Autodesk Inventor part; units mm, degrees
ref_plane "YZ Plane" through (0, 0, 0) normal (1, 0, 0) x (0, 1, 0)
ref_plane "XZ Plane" through (0, 0, 0) normal (0, 1, 0) x (-1, 0, 0)
ref_plane "XY Plane" through (0, 0, 0) normal (0, 0, 1) x (1, 0, 0)
sketch "Sketch1" plane through (0, 0, 0) normal (0, 1, 0) x (-1, 0, 0)
  line L0 (115, 92.5) -> (-115, 92.5)
  line L1 (-115, 92.5) -> (-115, -92.5)
  line L2 (-115, -92.5) -> (115, -92.5)
  line L3 (115, -92.5) -> (115, 92.5)
  point P0 (0, 0)
  dimension "d0" = 230
  dimension "d1" = 185
  dimension "d2" = 115
  dimension "d3" = 92.5
extrude "Extrusion1" add sketch "Sketch1" along normal blind 5
sketch "Sketch2" plane through (0, 0, 0) normal (0, -1, 0) x (1, 0, 0)
  line L0 (110, 87.5) -> (-110, 87.5)
  line L1 (-110, 87.5) -> (-110, -87.5)
  line L2 (-110, -87.5) -> (110, -87.5)
  line L3 (110, -87.5) -> (110, 87.5)
  line L4 (-115, 92.5) -> (115, 92.5)
  line L5 (-115, -92.5) -> (-115, 92.5)
  line L6 (115, -92.5) -> (-115, -92.5)
  line L7 (115, 92.5) -> (115, -92.5)
  line L8 (115, 92.5) -> (-115, 92.5)
  line L9 (-115, 92.5) -> (-115, -92.5)
  line L10 (-115, -92.5) -> (115, -92.5)
  line L11 (115, -92.5) -> (115, 92.5)
  point P0 (0, 0)
  dimension "d109" = 5
  dimension "d110" = 5
  dimension "d111" = 5
  dimension "d112" = 5
extrude "Extrusion2" add sketch "Sketch2" along normal blind 17.5
sketch "Sketch3" plane through (0, 5, 0) normal (0, 1, 0) x (1, 0, 0)
  circle A0 centre (-50, 0) radius 15.5
  point P0 (0, 0)
  dimension "d12" = 31
  dimension "d13" = 50
extrude "Extrusion3" cut sketch "Sketch3" against normal through all
sketch "Sketch4" plane through (0, 5, 0) normal (0, 1, 0) x (1, 0, 0)
  circle A0 centre (-50, 0) radius 15.5
  line L0 (-115, -92.5) -> (115, -92.5)
  line L1 (115, -92.5) -> (115, 92.5)
  line L2 (115, 92.5) -> (-115, 92.5)
  line L3 (-115, 92.5) -> (-115, -92.5)
  circle A1 centre (-97.5, -75) radius 7.5
  circle A2 centre (-97.5, 75) radius 7.5
  circle A3 centre (97.5, -75) radius 7.5
  circle A4 centre (97.5, 75) radius 7.5
  circle A5 centre (-97.5, -75) radius 8.5
  circle A6 centre (-97.5, 75) radius 8.5
  circle A7 centre (97.5, 75) radius 8.5
  circle A8 centre (97.5, -75) radius 8.5
  point P0 (0, 0)
  dimension "d16" = 15
  dimension "d17" = 17.5
  dimension "d18" = 17.5
  dimension "d19" = 15
  dimension "d20" = 15
  dimension "d21" = 15
  dimension "d22" = 17.5
  dimension "d23" = 17.5
  dimension "d24" = 17.5
  dimension "d25" = 17.5
  dimension "d26" = 17.5
  dimension "d27" = 17.5
  dimension "d28" = 17
  dimension "d29" = 17
  dimension "d30" = 17
  dimension "d31" = 17
  dimension "d34" = 75
  dimension "d35" = 97.5
extrude "Extrusion4" [suppressed]
sketch "Sketch8" plane through (0, 5, 0) normal (0, 1, 0) x (1, 0, 0)
  circle A0 centre (-50, 0) radius 15.5
  line L0 (-115, -92.5) -> (115, -92.5)
  line L1 (115, -92.5) -> (115, 92.5)
  line L2 (115, 92.5) -> (-115, 92.5)
  line L3 (-115, 92.5) -> (-115, -92.5)
  line L4 (-50, 13.5) -> (-50, -13.5)
  line L5 (-50, 13.5) -> (-115, 13.5)
  line L6 (-50, -13.5) -> (-115, -13.5)
  line L7 (-115, -13.5) -> (-115, 13.5)
  point P0 (0, 0)
  dimension "d51" = 27
  dimension "d52" = 13.5
  dimension "d62" = 31
extrude "Extrusion8" [suppressed]
sketch "Sketch10" plane through (-115, 5, -13.5) normal (0, 0, 1) x (1, 0, 0)
  line L0 (5, -20) -> (0, -20)
  line L1 (5, -5) -> (5, -20)
  line L2 (65, -5) -> (5, -5)
  line L3 (65, 0) -> (65, -5)
  line L4 (0, 0) -> (65, 0)
  line L5 (0, -20) -> (0, 0)
  line L6 (5, -17.5) -> (2.5, -17.5)
  line L7 (2.5, -17.5) -> (2.5, -2.5)
  line L8 (2.5, -2.5) -> (5, -2.5)
  line L9 (5, -2.5) -> (5, -17.5)
  line L10 (62.5, -5) -> (2.5, -5)
  line L11 (2.5, -5) -> (2.5, -2.5)
  line L12 (2.5, -2.5) -> (62.5, -2.5)
  line L13 (62.5, -2.5) -> (62.5, -5)
  point P0 (115, -5)
  dimension "d64" = 2.5
  dimension "d65" = 15
  dimension "d67" = 2.5
  dimension "d68" = 2.5
  dimension "d71" = 2.5
  dimension "d72" = 0
extrude "Extrusion10" [suppressed]
mirror "Mirror3" [suppressed]
sketch "Sketch12" plane through (0, 5, 0) normal (0, 1, 0) x (1, 0, 0)
  line L0 (-115, 13.5) -> (-110, 13.5)
  line L1 (-110, 13.5) -> (-110, 87.5)
  line L2 (-110, 87.5) -> (110, 87.5)
  line L3 (110, 87.5) -> (110, -87.5)
  line L4 (110, -87.5) -> (-110, -87.5)
  line L5 (-110, -87.5) -> (-110, -13.5)
  line L6 (-110, -13.5) -> (-115, -13.5)
  line L7 (-115, -13.5) -> (-115, -92.5)
  line L8 (-115, -92.5) -> (115, -92.5)
  line L9 (115, -92.5) -> (115, 92.5)
  line L10 (115, 92.5) -> (-115, 92.5)
  line L11 (-115, 92.5) -> (-115, 13.5)
  line L12 (-95.5, -92.5) -> (-85, -92.5)
  line L13 (-85, -92.5) -> (-85, -90)
  line L14 (-85, -90) -> (-95.5, -90)
  line L15 (-95.5, -90) -> (-95.5, -92.5)
  line L16 (85, -92.5) -> (95.5, -92.5)
  line L17 (95.5, -92.5) -> (95.5, -90)
  line L18 (95.5, -90) -> (85, -90)
  line L19 (85, -90) -> (85, -92.5)
  line L20 (-95.5, 92.5) -> (-85, 92.5)
  line L21 (-85, 92.5) -> (-85, 90)
  line L22 (-85, 90) -> (-95.5, 90)
  line L23 (-95.5, 90) -> (-95.5, 92.5)
  line L24 (85, 92.5) -> (95.5, 92.5)
  line L25 (95.5, 92.5) -> (95.5, 90)
  line L26 (95.5, 90) -> (85, 90)
  line L27 (85, 90) -> (85, 92.5)
  point P0 (0, 0)
  point P1 (0, 0)
  dimension "d87" = 10.5
  dimension "d88" = 2.5
  dimension "d90" = 10.5
  dimension "d91" = 2.5
  dimension "d93" = 2.5
  dimension "d94" = 10.5
  dimension "d96" = 2.5
  dimension "d97" = 10.5
  dimension "d114" = 85
  dimension "d115" = 85
  dimension "d116" = 85
  dimension "d117" = 85
  dimension "d122" = 5
  dimension "d123" = 5
  dimension "d124" = 230
  dimension "d125" = 230
  dimension "d126" = 19.5
  dimension "d127" = 19.5
  dimension "d128" = 19.5
  dimension "d129" = 19.5
  dimension "d131" = 5
extrude "Extrusion12" cut sketch "Sketch12" against normal blind 8 contours L10 L21 L22 L23 | L10 L25 L26 L27 | L8 L19 L18 L17 | L15 L14 L13 L8
sketch "Sketch13" plane through (0, -17.5, 0) normal (0, -1, 0) x (1, 0, 0)
  line L0 (-110, -87.5) -> (-110, 87.5)
  line L1 (-110, 87.5) -> (110, 87.5)
  line L2 (110, 87.5) -> (110, -87.5)
  line L3 (110, -87.5) -> (-110, -87.5)
  line L4 (-115, 92.5) -> (-115, -92.5)
  line L5 (-115, -92.5) -> (115, -92.5)
  line L6 (115, -92.5) -> (115, 92.5)
  line L7 (115, 92.5) -> (-115, 92.5)
  line L8 (112.75, -90.25) -> (-112.75, -90.25)
  line L9 (-112.75, -90.25) -> (-112.75, 90.25)
  line L10 (-112.75, 90.25) -> (112.75, 90.25)
  line L11 (112.75, 90.25) -> (112.75, -90.25)
  point P0 (0, 0)
  dimension "d101" = 185
  dimension "d102" = 180.5
  dimension "d104" = 225.5
  dimension "d105" = 112.75
  dimension "d106" = 90.25
extrude "Extrusion13" [suppressed]
fillet "Fillet1" radius 2 1 edges at (-65.5, 0, 0)
equation "\"d110\" = d109"
equation "\"d111\" = d109"
equation "\"d112\" = d109"
equation "\"d18\" = d17"
equation "\"d19\" = d16"
equation "\"d20\" = d16"
equation "\"d21\" = d16"
equation "\"d22\" = d17"
equation "\"d23\" = d22"
equation "\"d24\" = d17"
equation "\"d25\" = d24"
equation "\"d26\" = d17"
equation "\"d27\" = d26"
equation "\"d29\" = d28"
equation "\"d30\" = d28"
equation "\"d31\" = d28"
equation "\"d52\" = 0.5 * d51"
equation "\"d90\" = d87"
equation "\"d91\" = d88"
equation "\"d93\" = d88"
equation "\"d94\" = d87"
equation "\"d96\" = d88"
equation "\"d97\" = d87"
properties part number "Bottom Roof"
Geometry: final body of the model. Coordinates: model frame, mm. A direction names the side the tool comes from. Round coordinates to 2 decimals unless told otherwise and drop trailing zeros. Loops run counter-clockwise (first coordinate to the right, second up) from the corner with the lowest first, then second, coordinate; pieces in that order, holes last.
Q1. Section C-C on x = 42. Return loops of the section in (y, z).
Q2. Pull-direction query (Z, two-part tool) for faces 4 (the flat face through (2, 0, 1)), 5 (the flat face through (-115, -6, -1)), 6 (the flat face through (2, -6, -92.5)); classes: released by +Z, released by -Z, zero draft, split by the parting line, or undercut.
Q3. Pin query (flat end, axial travel): P1, Ø25, axis at x = -50, z = 0, coming from the +Y side; P2, Ø4, axis at x = -91.5, y = 3, coming from the -Z side; P3, Ø5, axis at x = 42, z = -46.5, coming from the -Y side; P4, Ø1.2, axis at x = -90, z = 91.5, coming from the +Y side. Return the tip coordinate at first contact, or that it passes through.
Q4. Section B-B on x = -50. Return loops of the section in (y, z), plus the area to 3 significant figures.
Q5. Section D-D on z = -32. Return loops of the section in (x, y), plus the area to 4 significant figures.
Q6. Access query for faces 1 (the flat face through (90, 1, -90)), 2 (the flat face through (2, -9, 87.5)), 3 (the flat face through (-90, 1, 90)). Directions: +Z, -Z, +X, -X, +Y, -Y. A direction counts if a zero-diameter tool reaches every point of the face in a straight line with its end or side. Return the directions, or none.
Q7. Material intervals for L1, parallel to X at y = 3.85, z = 0; L2, parallel to X at y = -0.25, z = 78; L3, parallel to Z at x = -50, y = 2.8, sorted ascending.
Q8. Section A-A on z = 0. Return loops of the section in (x, y).
Evaluation:
1. outline: (-17.5, -92.5) - (5, -92.5) - (5, 92.5) - (-17.5, 92.5) - (-17.5, 87.5) - (0, 87.5) - (0, -87.5) - (-17.5, -87.5) - close
2. face 4: undercut
2. face 5: zero draft
2. face 6: released by -Z
3. P1: passes through
3. P2: stops at z = -90
3. P3: stops at y = 0
3. P4: stops at y = -3
4. outline: (-17.5, -92.5) - (5, -92.5) - (5, -15.5) - (2, -15.5) arc R2 ccw to (0, -17.5) - (0, -87.5) - (-17.5, -87.5) - close; (-17.5, 87.5) - (0, 87.5) - (0, 17.5) arc R2 ccw to (2, 15.5) - (5, 15.5) - (5, 92.5) - (-17.5, 92.5) - close
4. area: 943 mm2
5. outline: (-115, -17.5) - (-110, -17.5) - (-110, 0) - (110, 0) - (110, -17.5) - (115, -17.5) - (115, 5) - (-115, 5) - close
5. area: 1,325 mm2
6. face 1: -Z, +Y
6. face 2: -Y
6. face 3: +Z, +Y
7. L1: x = -115 to -65.5, -34.5 to 115
7. L2: x = -115 to -110, 110 to 115
7. L3: z = -92.5 to -15.5, 15.5 to 92.5
8. outline: (-115, -17.5) - (-110, -17.5) - (-110, 0) - (-67.5, 0) arc R2 ccw to (-65.5, 2) - (-65.5, 5) - (-115, 5) - close; (-34.5, 2) arc R2 ccw to (-32.5, 0) - (110, 0) - (110, -17.5) - (115, -17.5) - (115, 5) - (-34.5, 5) - close
